Print and shaded views of the part. All mm, measured from the part's lowest x, y and z. A direction names the side the tool comes from. Round coordinates to 2 decimals unless told otherwise and drop trailing zeros. Write each loop counter-clockwise with the first axis right and the second up, starting at its lowest first coordinate (ties: lowest second). Pieces come first, ordered by that corner, then holes. Notation, with made-up numbers: (85.25, 33.5) - (107.25, 33.5) arc R33 cw to (107.25, 65.5) - close; hole circle Ø8 at (19.25, 8). An arc over 180 degrees is marked (long way). Put each result on its own line as item: value. Start each with the question number.
Item 1: Cut at D-D (z = 25). Give the cut face in (x, y).
Item 2: 3-axis set-ups, long thin cutter, end or side, ignore diameter. For the marked faces 1, 2 and 3: which of +Z, -Z, +X, -X, +Y, -Y reach the whole face in a straight line?
Item 3: Cut at C-C (y = 20). Give the cut face in (x, z), and give its area (3 significant figures).
Item 4: Drill centre lines: line 1 (Z direction, x = 6.75, y = 20.25); line 2 (Y direction, x = 9, z = 8.5); line 3 (Z direction, x = 9.25, y = 4). Where is each one in solid material? Low to high. Write a range as from..to.
Item 5: Pin check, flat tips, straight feed: pin 1 Ø2 at (x, y) = (4, 15.5) entering from -Z; pin 2 Ø1 at (y, z) = (8, 48) entering from -X; pin 3 Ø6 at (x, z) = (8, 72) entering from +Y. Stop position of each tip, or through.
Item 6: Cut at A-A (x = 5). Give the cut face in (y, z), and give its area (3 significant figures).
Item 7: Mould opens along Z. For the marked faces 4 and 5 say: released by +Z, released by -Z, zero draft, split by the parting line, or undercut.
Item 8: Cut at B-B (y = 5). Give the cut face in (x, z).
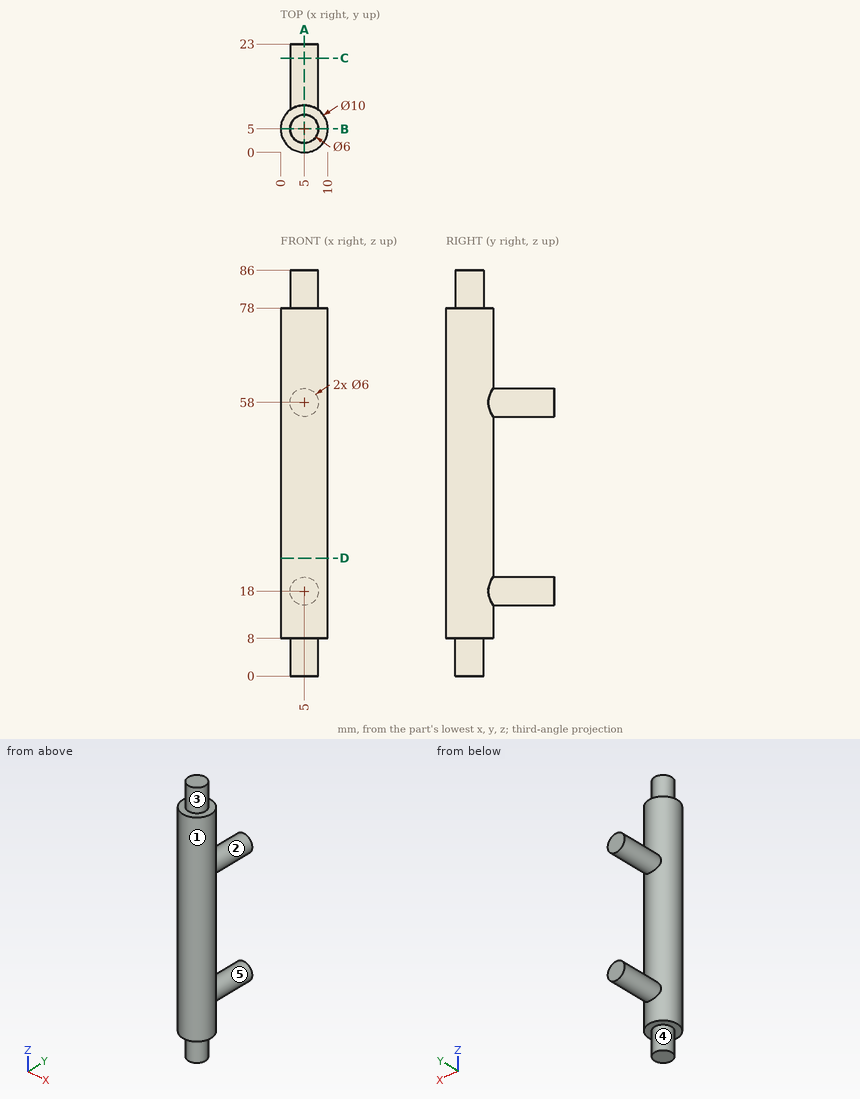
Output values:
1. outline: circle Ø10 at (5, 5)
2. face 1: none
2. face 2: +Y
2. face 3: +Z
3. outline: circle Ø6 at (5, 18); circle Ø6 at (5, 58)
3. area: 56.5 mm2
4. line 1: 15.56..20.44, 55.56..60.44
4. line 2: 2..8
4. line 3: 8..78
5. pin 1: z = 15
5. pin 2: x = 0.67
5. pin 3: y = 10
6. outline: (0, 8) - (2, 8) - (2, 0) - (8, 0) - (8, 8) - (10, 8) - (10, 15) - (23, 15) - (23, 21) - (10, 21) - (10, 55) - (23, 55) - (23, 61) - (10, 61) - (10, 78) - (8, 78) - (8, 86) - (2, 86) - (2, 78) - (0, 78) - close
6. area: 952 mm2
7. face 4: zero draft
7. face 5: undercut
8. outline: (0, 8) - (2, 8) - (2, 0) - (8, 0) - (8, 8) - (10, 8) - (10, 78) - (8, 78) - (8, 86) - (2, 86) - (2, 78) - (0, 78) - close
